Design review of the part shown in the three views and the two pictorial views. Dimensions are in mm from the part's minimum x, y and z. A direction names the side the tool comes from. Coordinates: 2 decimals unless noted, no trailing zeros. Write each loop counter-clockwise with the first axis right and the second up, starting at its lowest first coordinate (ties: lowest second). Pieces come first, ordered by that corner, then holes. Notation, with made-up numbers: M 88,-19.5 L 102,-19.5 A25 cw 102,11.5 Z; hole C 58,-12 d1. An arc over 180 degrees is marked long. One line per question, with ' | ' between items.
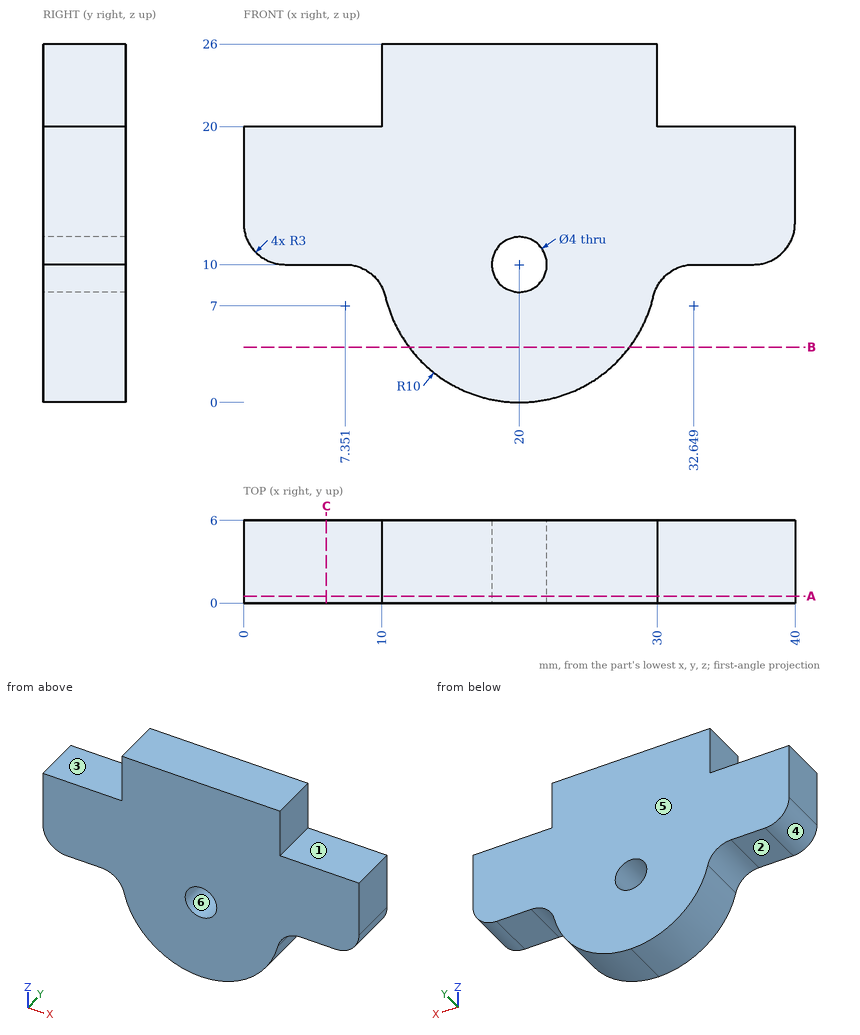
1. Take a section at B-B on z = 4. State the section outline as (x, y) points, plus the area to 3 significant figures.
Computed values:
outline: M 12,0 L 28,0 L 28,6 L 12,6 Z | area: 96.0 mm2
2. Clearance check with flat-ended pins moving along their axes: P1, Ø1.8, axis at x = 5, y = 3.5, coming from the +Z side; P2, Ø3.5, axis at x = 36, y = 4.5, coming from the -Z side. State where each tip first meets the part, or that it passes through.
Computed values:
P1: stops at z = 20 | P2: stops at z = 10
3. Take a section at C-C on x = 6. State the section outline as (y, z) points, plus the area to 3 significant figures.
Computed values:
outline: M 0,10 L 6,10 L 6,20 L 0,20 Z | area: 60.0 mm2
4. Machinability: for the marked faces 1, 2 and 3, which of the approach directions +Z, -Z, +X, -X, +Y, -Y give a long, thin tool a straight path to every point of the face, cutting with its end or side? Answer none if there is none.
Computed values:
face 1: +Z, +X, +Y, -Y | face 2: -Z, -X, +Y, -Y | face 3: +Z, -X, +Y, -Y
5. For line 1 along Z through (x, y) = (20, 3.8); line 2 along Z through (x, y) = (35, 2.7); line 3 along X through (y, z) = (3.9, 22.25), list the stretches that pass through material, from the lowest coordinate up.
Computed values:
line 1: z = 0 to 8, 12 to 26 | line 2: z = 10 to 20 | line 3: x = 10 to 30
6. Take a section at A-A on y = 0.5. State the section outline as (x, z) points, plus the area to 3 significant figures.
Computed values:
outline: M 0,13 A3 ccw 3,10 L 7.35,10 A3 cw 10.27,7.69 A10 ccw 20,0 A10 ccw 29.73,7.69 A3 cw 32.65,10 L 37,10 A3 ccw 40,13 L 40,20 L 30,20 L 30,26 L 10,26 L 10,20 L 0,20 Z; hole C 20,10 d4 | area: 663 mm2
7. Draft analysis for pull direction Z (two halves, no side actions). For the marked faces 4, 5 and 6, state which applies: pulls with the +Z half, pulls with the -Z half, needs draft (parallel to the pull), parting line crosses it, or undercut.
Computed values:
face 4: pulls with the -Z half | face 5: needs draft | face 6: undercut
